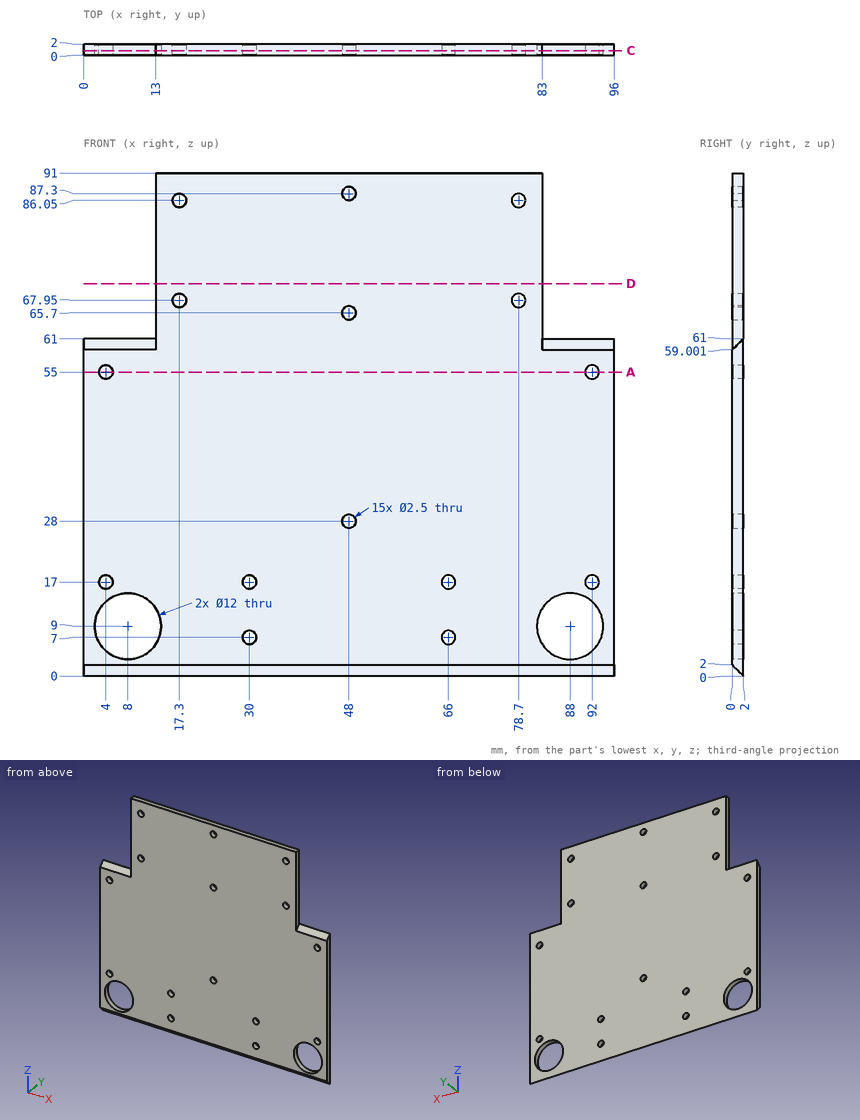
Part print with two shaded views. Sizes in mm from the minimum x, y, z corner. Give positions to 0.01 mm unless a question says otherwise; leave off trailing zeros. Loops run counter-clockwise (first coordinate to the right, second up) from the corner with the lowest first, then second, coordinate; pieces in that order, holes last. Notation, with made-up numbers: (-17.5, -27.5) -> (15.5, -27.5) arc R34 ccw to (15.5, 7.5) -> close; hole circle Ø8 at (88.25, 15.5). An arc over 180 degrees is marked (long way). One line per question, with ' | ' between items.
Q1. Cut at D-D, the plane z = 71. Write the cut outline in (x, y), plus the area to 3 significant figures.
Filled sheet:
outline: (13, 0) -> (83, 0) -> (83, 2) -> (13, 2) -> close | area: 140 mm²
Q2. Drill centre lines: line 1 along X through (y, z) = (0.6, 86); line 2 along X through (y, z) = (1.2, 69) (1 decimal); line 3 along X through (y, z) = (1.2, 18). Where is each one in solid material? Low to high. Write a range as [from, to].
Filled sheet:
line 1: x = [13, 16.05], [18.55, 77.45], [79.95, 83] | line 2: x = [13, 16.6], [18, 78], [79.4, 83] | line 3: x = [0, 3.25], [4.75, 29.25], [30.75, 65.25], [66.75, 91.25], [92.75, 96]
Q3. Cut at A-A, the plane z = 55. Write the cut outline in (x, y).
Filled sheet:
outline: (0, 0) -> (2.75, 0) -> (2.75, 2) -> (0, 2) -> close; (5.25, 0) -> (90.75, 0) -> (90.75, 2) -> (5.25, 2) -> close; (93.25, 0) -> (96, 0) -> (96, 2) -> (93.25, 2) -> close
Q4. Drop flat-ended pins along their axis: pin 1 (0.6 mm diameter, centred on y = 1.5, z = 71.5, fed in from -X); pin 2 (1 mm diameter, centred on x = 51, y = 1, fed in from -Z). Give the stop position or say it passes through.
Filled sheet:
pin 1: stops at x = 13 | pin 2: stops at z = 0.5
Q5. Cut at C-C, the plane y = 0.8. Count the separate pieces of the cut face and the enclosed holes in it, plus the area to 3 significant figures.
Filled sheet:
separate pieces: 1 | enclosed holes: 17 | area: 7,510 mm²
